The listing builds one solid part. Answer for the finished solid, in the listing's coordinates (mm). A direction names the side the tool comes from. Round coordinates to 2 decimals unless told otherwise and drop trailing zeros. Loops run counter-clockwise (first coordinate to the right, second up) from the corner with the lowest first, then second, coordinate; pieces in that order, holes last. Notation, with made-up numbers: (-28.75, 56.25) -> (-16.75, 56.25) arc R29 cw to (-16.75, 81.25) -> close; hole circle Ø4 at (-18.75, -4.75). An arc over 180 degrees is marked (long way). One line per question, with ' | ' between items.
from build123d import *

# Parameters (mm, degrees)
F0_W     = 870
F0_H     = 890
F1_DEPTH = 1070
F2_W     = 530
F2_H     = 540
F3_DEPTH = 560
F4_W     = 180
F4_H     = 310
F5_DEPTH = 560


with BuildPart() as f1:
    # F0 (on Top) → F1 (new body)
    with BuildSketch(Plane.XY):
        Rectangle(F0_W, F0_H)
    extrude(amount=F1_DEPTH)

    # F2 (on face) → F3 (cut)
    with BuildSketch(Plane(origin=(-435, 0, 0), x_dir=(0, -1, 0), z_dir=(-1, 0, 0))):
        with Locations((0, 800)):
            Rectangle(F2_W, F2_H)
    extrude(amount=-F3_DEPTH, mode=Mode.SUBTRACT)

    # F4 (on face) → F5 (cut, through all)
    with BuildSketch(Plane(origin=(-435, 0, 0), x_dir=(0, -1, 0), z_dir=(-1, 0, 0))):
        with Locations((-355, 915)):
            Rectangle(F4_W, F4_H)
        with Locations((355, 915)):
            Rectangle(F4_W, F4_H)
    extrude(amount=-F5_DEPTH, mode=Mode.SUBTRACT)


solid = f1.part
Q1. A cutting plane is placed at C-C on z = 643.5. Give the vertices of the cut face in (x, y), plus the area to 4 significant figures.
Numbers:
outline: (-435, -445) -> (435, -445) -> (435, 445) -> (-435, 445) -> (-435, 265) -> (125, 265) -> (125, -265) -> (-435, -265) -> close | area: 477,500 mm^2
Q2. Given pin 1 Ø2 at (x, y) = (113, -326) entering from +Z, flat-ended and moving along its own axis, determine where the tip first touches the part or whether it passes through.
Numbers:
pin 1: z = 760
Q3. A cutting plane is placed at A-A on x = 59.5. Give the vertices of the cut face in (y, z), plus the area to 4 significant figures.
Numbers:
outline: (-445, 0) -> (445, 0) -> (445, 760) -> (265, 760) -> (265, 530) -> (-265, 530) -> (-265, 760) -> (-445, 760) -> close | area: 554,500 mm^2
Q4. For faces 1 (the face through (435, -6, 528)), 2 (the face through (-159, 265, 643)), 3 (the face through (-159, 356, 760)), determine the directions among +Z, -Z, +X, -X, +Y, -Y from which every point of the face is accessible in a straight line to the end or side of a thin tool.
Numbers:
face 1: +Z, -Z, +X, +Y, -Y | face 2: +Z, -X | face 3: +Z, -X, +Y, -Y
Q5. Find the intervals of material crossed by line 1 (Y direction, x = -311.5, z = 598); line 2 (Z direction, x = -387, y = -140); line 3 (X direction, y = 198.5, z = 706), in increasing order. Write a range as from..to.
Numbers:
line 1: -445..-265, 265..445 | line 2: 0..530 | line 3: 125..435
Q6. A cutting plane is placed at B-B on y = -376.5. Give the vertices of the cut face in (x, z), plus the area to 3 significant figures.
Numbers:
outline: (-435, 0) -> (435, 0) -> (435, 1070) -> (125, 1070) -> (125, 760) -> (-435, 760) -> close | area: 757,000 mm^2
Q7. A cutting plane is placed at D-D on y = -20. Give the vertices of the cut face in (x, z).
Numbers:
outline: (-435, 0) -> (435, 0) -> (435, 1070) -> (125, 1070) -> (125, 530) -> (-435, 530) -> close
